from build123d import *

# Parameters (mm, degrees)
SKETCH1_W      = 12.1
SKETCH1_H      = 15.5
EXTRUDE1_DEPTH = 6.7
SKETCH5_W      = 13
SKETCH5_H      = 1.3
EXTRUDE5_DEPTH = 6.4
SKETCH6_W      = 0.6
SKETCH6_H      = 2.3
EXTRUDE6_DEPTH = 0.1
SKETCH7_R      = 3
EXTRUDE7_DEPTH = 22


with BuildPart() as part:
    # Sketch1 → Extrude1 (new body)
    with BuildSketch(Plane(origin=(0, 0, 0), x_dir=(1, 0, 0), z_dir=(0, 1, 0))):
        with Locations((0, -0.95)):
            Rectangle(SKETCH1_W, SKETCH1_H)
    extrude(amount=EXTRUDE1_DEPTH)

    # Sketch5 → Extrude5 (add)
    with BuildSketch(Plane(origin=(0, 0, 0), x_dir=(1, 0, 0), z_dir=(0, 1, 0))):
        with Locations((0, -8.05)):
            Rectangle(SKETCH5_W, SKETCH5_H)
    extrude(amount=EXTRUDE5_DEPTH)

    # Sketch6 → Extrude6 (add)
    with BuildSketch(Plane(origin=(0, 0, 0), x_dir=(1, 0, 0), z_dir=(0, 1, 0))):
        with Locations((-1, -9.85)):
            Rectangle(SKETCH6_W, SKETCH6_H)
        with Locations((-3, -9.85)):
            Rectangle(SKETCH6_W, SKETCH6_H)
        with Locations((-5, -9.85)):
            Rectangle(SKETCH6_W, SKETCH6_H)
        with Locations((5, -9.85)):
            Rectangle(SKETCH6_W, SKETCH6_H)
        with Locations((3, -9.85)):
            Rectangle(SKETCH6_W, SKETCH6_H)
        with Locations((1, -9.85)):
            Rectangle(SKETCH6_W, SKETCH6_H)
    extrude(amount=EXTRUDE6_DEPTH)

    # Sketch7 → Extrude7 (add)
    with BuildSketch(Plane(origin=(0, 6.7, 0), x_dir=(1, 0, 0), z_dir=(0, 1, 0))):
        with Locations(Location((0, 0, 0), (0, 0, 270))):
            Circle(SKETCH7_R)
    extrude(amount=EXTRUDE7_DEPTH)


solid = part.part
For this review, take the finished solid that the model builds, in its own axes (mm). A direction names the side the tool comes from. Round coordinates to 2 decimals unless told otherwise and drop trailing zeros. Order: outer loops, then holes, each group sorted by start corner. A loop starts at its lowest first (then second) coordinate and runs counter-clockwise, first axis right, second up. Notation, with made-up numbers: (48.5, 10) -> (71.5, 10) arc R15 ccw to (71.5, 24) -> close; hole circle Ø8 at (-27, 6). An arc over 180 degrees is marked (long way). Put each result on its own line as item: value.
Q1. Add section C-C on y = 15. Write out the cut boundary in (x, z).
Check result:
outline: circle Ø6 at (0, 0)
Q2. For probe 1 along Y at (x, z) = (-4.5, 0.5); probe 2 along Z at (x, y) = (2.75, 6); probe 3 along X at (y, z) = (6.25, -2.25), list the stretches that pass through material, from the lowest coordinate up. Write a range as [from, to].
Check result:
probe 1: [0, 6.7]
probe 2: [-6.8, 8.7]
probe 3: [-6.05, 6.05]
Q3. Add section D-D on x = 2.25. Write out the cut boundary in (y, z).
Check result:
outline: (0, -6.8) -> (6.7, -6.8) -> (6.7, -1.98) -> (28.7, -1.98) -> (28.7, 1.98) -> (6.7, 1.98) -> (6.7, 8.7) -> (0, 8.7) -> close
Q4. Add section A-A on z = 0. Write out the cut boundary in (x, y), plus the area to 3 significant figures.
Check result:
outline: (-6.05, 0) -> (6.05, 0) -> (6.05, 6.7) -> (3, 6.7) -> (3, 28.7) -> (-3, 28.7) -> (-3, 6.7) -> (-6.05, 6.7) -> close
area: 213 mm2
Q5. Machinability: for faces 1 (the flat face through (6.5, 3, 8)), 2 (the cylindrical face through (0.9, 17.55, 2.86)), which of the approach directions +Z, -Z, +X, -X, +Y, -Y give a long, thin tool a straight path to every point of the face, cutting with its end or side? Answer none if there is none.
Check result:
face 1: +Z, -Z, +X, +Y, -Y
face 2: +Y
Q6. Add section B-B on x = -5. Write out the cut boundary in (y, z), plus the area to 3 significant figures.
Check result:
outline: (0, -6.8) -> (6.7, -6.8) -> (6.7, 8.7) -> (0.1, 8.7) -> (0.1, 11) -> (0, 11) -> close
area: 104 mm2
Q7. Insertion check: pin 1 Ø2 at (x, z) = (0, 6.5) entering from -Y; pin 2 Ø5.5 at (y, z) = (2, 0.5) entering from +X; pin 3 Ø1.5 at (y, z) = (7.5, 0) entering from +X; pin 4 Ø0.7 at (x, z) = (3, 9.5) entering from +Y. Each pin has a flat end and moves straight along its axis. Give the tip position at first contact, or say it passes through.
Check result:
pin 1: y = 0
pin 2: x = 6.05
pin 3: x = 3
pin 4: y = 0.1
